Geometry check sheet. Reference: the model listing, model coordinates, mm. A direction names the side the tool comes from. Give positions to 0.01 mm unless a question says otherwise; leave off trailing zeros. Loops run counter-clockwise (first coordinate to the right, second up) from the corner with the lowest first, then second, coordinate; pieces in that order, holes last. Notation, with made-up numbers: (36, -33.75) -> (85, -33.75) arc R26 ccw to (85, -6.75) -> close; hole circle Ø5 at (16.5, 79.25). An arc over 180 degrees is marked (long way). One line per item, written item: value. Start each with the question number.
(1) Tool access check on faces 1 (the face through (-0.74, 3.35, 1.8)), 2 (the face through (0, 1.786, 3)), 3 (the face through (-0.05, -2.24, 0)). Record the directions out of +Z, -Z, +X, -X, +Y, -Y that give a thin tool (end or side, any length) a straight path to the whole face; none if there is none.
(2) Gauge pin test, flat ends, axial feed: pin 1 Ø1.8 at (x, y) = (-0.5, 0) entering from +Z; pin 2 Ø4 at (x, z) = (0.5, -14.5) entering from +Y; pin 3 Ø0.6 at (x, z) = (0.5, 3.5) entering from +Y. Record the tip position at first contact, or that the pin passes through.
(3) Sectioned sample at A-A, the plane x = 0. Record the cut outline in (y, z) (3 decimals), then the cut area to 3 significant figures.
(4) Draft check along Y on faces 4 (the face through (-1.987, -0.626, -20.098)), 5 (the face through (1.554, -0.88, 3.164)), 6 (the face through (0, 0, -41.275)). Enter one of: pulls with the +Y half, pulls with the -Y half, needs draft (parallel to the pull), parting line crosses it, or undercut.
(5) Scan lines: line 1 along Z through (x, y) = (-0.25, 1.25) (3 decimals); line 2 along Z through (x, y) = (0.75, -2); line 3 along Y through (x, z) = (0.75, 2). Record each from-to range of solid material in increasing order. Write a range as from..to.
(6) Sectioned sample at B-B, the plane z = -3.5. Record the cut outline in (x, y), then the cut area to 3 significant figures.
Autodesk Inventor part; units mm, degrees
ref_plane "YZ Plane" through (0, 0, 0) normal (1, 0, 0) x (0, 1, 0)
ref_plane "XZ Plane" through (0, 0, 0) normal (0, 1, 0) x (-1, 0, 0)
ref_plane "XY Plane" through (0, 0, 0) normal (0, 0, 1) x (1, 0, 0)
sketch "Sketch1" plane through (0, 0, 0) normal (0, 0, 1) x (1, 0, 0)
  circle A0 centre (0, 0) radius 3.429
  dimension "d0" = 6.858
extrude "Extrusion1" add sketch "Sketch1" along normal blind 4.1656
sketch "Sketch2" plane through (0, 0, 0) normal (0, 0, -1) x (-1, 0, 0)
  circle A0 centre (0, 0) radius 3.429
  circle A1 centre (0, 0) radius 2.0828
  dimension "d3" = 4.1656
extrude "Extrusion2" add sketch "Sketch2" along normal blind 41.275 contours A1
sketch "Sketch3" plane through (0, 0, 4.1656) normal (0, 0, 1) x (1, 0, 0)
  circle A0 centre (0, 0) radius 3.429
  line L0 (-1.0311, 1.7859) -> (1.0311, 1.7859)
  line L1 (1.0311, 1.7859) -> (2.0622, 0)
  line L2 (2.0622, 0) -> (1.0311, -1.7859)
  line L3 (1.0311, -1.7859) -> (-1.0311, -1.7859)
  line L4 (-1.0311, -1.7859) -> (-2.0622, 0)
  line L5 (-2.0622, 0) -> (-1.0311, 1.7859)
  dimension "d6" = 3.5719
extrude "Extrusion3" cut sketch "Sketch3" against normal blind 2.032 contours L0 L1 L2 L3 L4 L5
thread "Thread1"
chamfer "Chamfer1" distance 0.508 angle 45 1 edges at (2.0828, 0, -41.275)
chamfer "Chamfer2" distance 0.508 angle 45 1 edges at (-3.429, 0, 4.1656)
properties part number "10-32 x1000" material "Steel"
Calculated:
1. face 1: +Z, -Z
1. face 2: +Z
1. face 3: -Z
2. pin 1: stops at z = 2.13
2. pin 2: stops at y = 2.08
2. pin 3: stops at y = 3.42
3. outline: (-3.429, 0) -> (-2.083, 0) -> (-2.083, -40.767) -> (-1.575, -41.275) -> (1.575, -41.275) -> (2.083, -40.767) -> (2.083, 0) -> (3.429, 0) -> (3.429, 3.658) -> (2.921, 4.166) -> (1.786, 4.166) -> (1.786, 2.134) -> (-1.786, 2.134) -> (-1.786, 4.166) -> (-2.921, 4.166) -> (-3.429, 3.658) -> close
3. area: 193 mm2
4. face 4: parting line crosses it
4. face 5: undercut
4. face 6: needs draft
5. line 1: z = -41.275..2.134
5. line 2: z = 0..4.17
5. line 3: y = -3.35..3.35
6. outline: circle Ø4.17 at (0, 0)
6. area: 13.6 mm2
